Answer from the drawing. Dimensions are ordinates in mm from the lowest x, y and z of the part. A direction names the side the tool comes from. Round coordinates to 2 decimals unless told otherwise and drop trailing zeros. Loops run counter-clockwise (first coordinate to the right, second up) from the corner with the lowest first, then second, coordinate; pieces in that order, holes last.
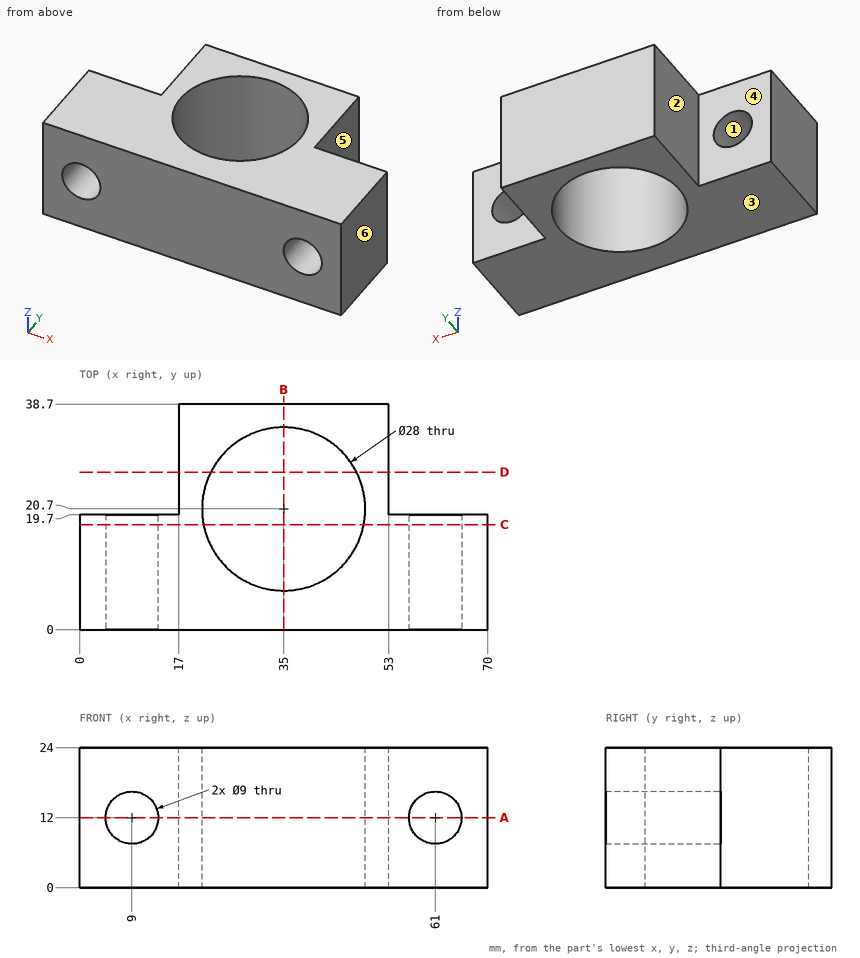
1. Find section A-A (z = 12). Write down the section's boundary in (x, y).
Answer key:
outline: (0, 0) - (4.5, 0) - (4.5, 19.7) - (0, 19.7) - close; (13.5, 0) - (56.5, 0) - (56.5, 19.7) - (53, 19.7) - (53, 38.7) - (17, 38.7) - (17, 19.7) - (13.5, 19.7) - close; (65.5, 0) - (70, 0) - (70, 19.7) - (65.5, 19.7) - close; hole circle Ø28 at (35, 20.7)
2. Find section C-C (y = 18). Write down the section's boundary in (x, z), then the cut area to 3 significant figures.
Answer key:
outline: (0, 0) - (21.26, 0) - (21.26, 24) - (0, 24) - close; (48.74, 0) - (70, 0) - (70, 24) - (48.74, 24) - close; hole circle Ø9 at (9, 12); hole circle Ø9 at (61, 12)
area: 893 mm2
3. Which of the six approach directions +Z, -Z, +X, -X, +Y, -Y give full straight-line access (tool end or side, diameter ignored) to the marked faces 4, 5 and 6?
Answer key:
face 4: +Z, -Z, -X, +Y
face 5: +Z, -Z, +X, +Y
face 6: +Z, -Z, +X, +Y, -Y
4. Consider probe 1 along Y at (x, z) = (35, 14); probe 2 along Z at (x, y) = (61, 8); probe 3 along X at (y, z) = (26, 10.5). Determine where each line is inside the solid, lowest interval first.
Answer key:
probe 1: y = 0 to 6.7, 34.7 to 38.7
probe 2: z = 0 to 7.5, 16.5 to 24
probe 3: x = 17 to 22.04, 47.96 to 53
5. Determine the mould class of the marked faces 1, 2 and 3 for opening direction Z: +Z half, -Z half, draft (parallel to the pull), parting line (faces both ways), or undercut.
Answer key:
face 1: undercut
face 2: draft
face 3: -Z half
6. Find section D-D (y = 27). Write down the section's boundary in (x, z).
Answer key:
outline: (17, 0) - (22.5, 0) - (22.5, 24) - (17, 24) - close; (47.5, 0) - (53, 0) - (53, 24) - (47.5, 24) - close
7. Given pin 1 (1.5 mm diameter, centred on x = 43.5, y = 9, fed in from -Z); pin 2 (8.5 mm diameter, centred on x = 62.5, z = 7, fed in from +Y), each flat-ended and moving along its own axis, determine where each tip first touches the part or whether it passes through.
Answer key:
pin 1: stops at z = 0
pin 2: stops at y = 19.7
8. Find section B-B (x = 35). Write down the section's boundary in (y, z).
Answer key:
outline: (0, 0) - (6.7, 0) - (6.7, 24) - (0, 24) - close; (34.7, 0) - (38.7, 0) - (38.7, 24) - (34.7, 24) - close
